```python
from build123d import *

# Parameters (mm, degrees)
F1_DEPTH = 2
F2_DEPTH = 4


with BuildPart() as f1:
    # F0 (on Top) → F1 (new body)
    with BuildSketch(Plane.XY):
        with BuildLine():
            ThreePointArc((18.0739206718, 6.0497422268), (13.5205869532, 7.4719650911), (8.9672532347, 6.0497422268))
            Line((8.9672532347, 6.0497422268), (18.0739206718, 6.0497422268))
        make_face()
        with BuildLine():
            Line((18.0739206718, 6.0497422268), (8.9672532347, 6.0497422268))
            ThreePointArc((8.9672532347, 6.0497422268), (2.8913578077, 3.8979685049), (-3.5327467653, 3.3711707982))
            Line((-3.5327467653, 3.3711707982), (-3.5327467653, -1.4502577732))
            Line((-3.5327467653, -1.4502577732), (21.4672532347, -1.4502577732))
            Line((21.4672532347, -1.4502577732), (21.4672532347, 0.3941879553))
            ThreePointArc((21.4672532347, 0.3941879553), (20.3805303589, 3.5879311345), (18.0739206718, 6.0497422268))
        make_face()
        with BuildLine():
            Line((-3.5327467653, -1.4502577732), (-3.5327467653, 3.3711707982))
            ThreePointArc((-3.5327467653, 3.3711707982), (-9.9568513384, 3.8979685049), (-16.0327467653, 6.0497422268))
            Line((-16.0327467653, 6.0497422268), (-25.1394142025, 6.0497422268))
            ThreePointArc((-25.1394142025, 6.0497422268), (-27.4460238896, 3.5879311345), (-28.5327467653, 0.3941879553))
            Line((-28.5327467653, 0.3941879553), (-28.5327467653, -1.4502577732))
            Line((-28.5327467653, -1.4502577732), (-22.9360804839, -1.4502577732))
            ThreePointArc((-22.9360804839, -1.4502577732), (-20.5860804839, 0.8997422268), (-18.2360804839, -1.4502577732))
            Line((-18.2360804839, -1.4502577732), (-3.5327467653, -1.4502577732))
        make_face()
        with BuildLine():
            Line((-25.1394142025, 6.0497422268), (-16.0327467653, 6.0497422268))
            ThreePointArc((-16.0327467653, 6.0497422268), (-20.5860804839, 7.4719650911), (-25.1394142025, 6.0497422268))
        make_face()
        with BuildLine():
            ThreePointArc((21.4672532347, -1.4502577732), (21.5205869532, -0.5280349089), (21.4672532347, 0.3941879553))
            Line((21.4672532347, 0.3941879553), (21.4672532347, -1.4502577732))
        make_face()
        with BuildLine():
            Line((21.4672532347, -1.4502577732), (-3.5327467653, -1.4502577732))
            Line((-3.5327467653, -1.4502577732), (-3.5327467653, -6.2716863446))
            ThreePointArc((-3.5327467653, -6.2716863446), (2.8913578077, -6.7984840513), (8.9672532347, -8.9502577732))
            Line((8.9672532347, -8.9502577732), (18.0739206718, -8.9502577732))
            ThreePointArc((18.0739206718, -8.9502577732), (20.3805303589, -6.4884466809), (21.4672532347, -3.2947035017))
            Line((21.4672532347, -3.2947035017), (21.4672532347, -1.4502577732))
        make_face()
        with BuildLine():
            Line((-3.5327467653, -6.2716863446), (-3.5327467653, -1.4502577732))
            Line((-3.5327467653, -1.4502577732), (-18.2360804839, -1.4502577732))
            ThreePointArc((-18.2360804839, -1.4502577732), (-20.5860804839, -3.8002577732), (-22.9360804839, -1.4502577732))
            Line((-22.9360804839, -1.4502577732), (-28.5327467653, -1.4502577732))
            Line((-28.5327467653, -1.4502577732), (-28.5327467653, -3.2947035017))
            ThreePointArc((-28.5327467653, -3.2947035017), (-27.4460238896, -6.4884466809), (-25.1394142025, -8.9502577732))
            Line((-25.1394142025, -8.9502577732), (-16.0327467653, -8.9502577732))
            ThreePointArc((-16.0327467653, -8.9502577732), (-9.9568513384, -6.7984840513), (-3.5327467653, -6.2716863446))
        make_face()
        with BuildLine():
            ThreePointArc((21.4672532347, -3.2947035017), (21.5205869532, -2.3724806375), (21.4672532347, -1.4502577732))
            Line((21.4672532347, -1.4502577732), (21.4672532347, -3.2947035017))
        make_face()
        with BuildLine():
            Line((-28.5327467653, -1.4502577732), (-28.5327467653, 0.3941879553))
            ThreePointArc((-28.5327467653, 0.3941879553), (-28.5860804839, -0.5280349089), (-28.5327467653, -1.4502577732))
        make_face()
        with BuildLine():
            ThreePointArc((-25.1394142025, -8.9502577732), (-20.5860804839, -10.3724806375), (-16.0327467653, -8.9502577732))
            Line((-16.0327467653, -8.9502577732), (-25.1394142025, -8.9502577732))
        make_face()
        with BuildLine():
            Line((18.0739206718, -8.9502577732), (8.9672532347, -8.9502577732))
            ThreePointArc((8.9672532347, -8.9502577732), (13.5205869532, -10.3724806375), (18.0739206718, -8.9502577732))
        make_face()
        with BuildLine():
            Line((-28.5327467653, -3.2947035017), (-28.5327467653, -1.4502577732))
            ThreePointArc((-28.5327467653, -1.4502577732), (-28.5860804839, -2.3724806375), (-28.5327467653, -3.2947035017))
        make_face()
    extrude(amount=F1_DEPTH)

    # F0 (on Top) → F2 (join)
    with BuildSketch(Plane.XY):
        with BuildLine():
            ThreePointArc((-22.9360804839, -1.4502577732), (-20.5860804839, -3.8002577732), (-18.2360804839, -1.4502577732))
            Line((-18.2360804839, -1.4502577732), (-20.5860804839, -1.4502577732))
            Line((-20.5860804839, -1.4502577732), (-22.9360804839, -1.4502577732))
        make_face()
        with BuildLine():
            Line((-20.5860804839, -1.4502577732), (-18.2360804839, -1.4502577732))
            ThreePointArc((-18.2360804839, -1.4502577732), (-20.5860804839, 0.8997422268), (-22.9360804839, -1.4502577732))
            Line((-22.9360804839, -1.4502577732), (-20.5860804839, -1.4502577732))
        make_face()
    extrude(amount=F2_DEPTH)


solid = f1.part
```
Can you work these out from the model? Positions are in its coordinate system, mm. A direction names the side the tool comes from. Give positions to 0.01 mm unless a question says otherwise; leave off trailing zeros. Loops run counter-clockwise (first coordinate to the right, second up) from the corner with the lowest first, then second, coordinate; pieces in that order, holes last. Notation, with made-up numbers: M 36,81.5 L 81,81.5 A13 cw 81,99.5 Z; hole C -6.5,-38 d2. An arc over 180 degrees is marked long. Use one line per item in the form item = value. Start each with the question number.
(1) I want a section at C-C, the plane z = 0.95. Write out the boundary of the cut face in (x, y), and give its area (3 significant figures).
(2) I'm going to push flat-ended pins straight in: P1, Ø2, axis at y = 5, z = 0.5, coming from the -X side; P2, Ø1.5, axis at x = 9, y = -4, coming from the -Z side; P3, Ø5.5, axis at x = -8.5, y = -4.5, coming from the +Z side; P4, Ø1, axis at y = -8, z = 2, coming from the -X side. Where does each tip first touch, or does it pass through?
(3) Please list where these lines run through material, in increasing order: line 1 (Z direction, x = -14.5, y = -4); line 2 (Y direction, x = -2.5, z = 1.1); line 3 (Y direction, x = 15, z = 1.9).
(4) On a 3-axis mill with a long thin cutter (end or side, diameter ignored), from which of +Z, -Z, +X, -X, +Y, -Y can I reach the whole of each face in a straight line? I mean faces 4 (the flat face through (-21, -1, 4)), 5 (the cylindrical face through (2.8, -6.78, 0.99)), 6 (the cylindrical face through (2.98, 3.917, 0.986)). Say none if no direction works.
(5) I want a section at A-A, the plane y = 5. Write out the boundary of the cut face in (x, z).
(6) I want a section at D-D, the plane y = -1. Write out the boundary of the cut face in (x, z), and give its area (3 significant figures).
(7) I want a section at B-B, the plane x = -20. Write out the boundary of the cut face in (y, z).
(8) Thinking about a two-plate mould opening in X: for faces 1 (the cylindrical face through (-10.05, -6.82, 0.99)), 2 (the cylindrical face through (-22.45, -2.88, 2.99)), 3 (the flat face through (-4, -1, 0)), which applies, released by +X, released by -X, zero draft, split by the parting line, or undercut?
Worked out:
q1.outline = M -28.53,-1.45 A8 ccw -16.03,-8.95 A25 cw -3.53,-6.27 A25 cw 8.97,-8.95 A8 ccw 21.47,-1.45 A8 ccw 8.97,6.05 A25 cw -3.53,3.37 A25 cw -16.03,6.05 A8 ccw Z
q1.area = 664 mm²
q2.P1 = -27.18
q2.P2 = 0
q2.P3 = 2
q2.P4 = -26.73
q3.line_1 = 0 to 2
q3.line_2 = -6.24 to 3.34
q3.line_3 = -10.23 to 7.33
q4.face_4 = +Z, +X, -X, +Y, -Y
q4.face_5 = +Z, -Z, -Y
q4.face_6 = +Z, -Z, +Y
q5.outline = M -26.37,0 L -13.67,0 L -13.67,2 L -26.37,2 Z; M 6.6,0 L 19.3,0 L 19.3,2 L 6.6,2 Z
q6.outline = M -28.57,0 L 21.51,0 L 21.51,2 L -18.28,2 L -18.28,4 L -22.89,4 L -22.89,2 L -28.57,2 Z
q6.area = 109 mm²
q7.outline = M -10.35,0 L 7.45,0 L 7.45,2 L 0.83,2 L 0.83,4 L -3.73,4 L -3.73,2 L -10.35,2 Z
q8.face_1 = undercut
q8.face_2 = split by the parting line
q8.face_3 = zero draft
